Geometry check sheet. Reference: the model listing, model coordinates, mm. Face numbers are marked on the shaded views. A direction names the side the tool comes from. Give positions to 0.01 mm unless a question says otherwise; leave off trailing zeros. Loops run counter-clockwise (first coordinate to the right, second up) from the corner with the lowest first, then second, coordinate; pieces in that order, holes last. Notation, with made-up numbers: (87, 18) -> (122, 18) arc R22 cw to (122, 49) -> close; hole circle Ø10 at (-3.5, -32). An arc over 180 degrees is marked (long way). One line per question, with ' | ' between items.
from build123d import *

# Parameters (mm, degrees)
F0_R     = 1.5
F1_DEPTH = 8
F2_W     = 14.905
F2_H     = 7.65
F3_DEPTH = 7.001
F4_W     = 10.16
F4_H     = 12.091013
F5_DEPTH = 8.351


with BuildPart() as f1:
    # F0 (on Front) → F1 (new body, symmetric)
    with BuildSketch(Plane.XZ):
        with BuildLine():
            Line((9.825, 3.5), (-9.825, 3.5))
            ThreePointArc((-9.825, 3.5), (-13.325, 0), (-9.825, -3.5))
            Line((-9.825, -3.5), (9.825, -3.5))
            ThreePointArc((9.825, -3.5), (13.325, 0), (9.825, 3.5))
        make_face()
        with Locations((-9.825, 0)):
            Circle(F0_R, mode=Mode.SUBTRACT)
        with Locations((9.825, 0)):
            Circle(F0_R, mode=Mode.SUBTRACT)
    extrude(amount=F1_DEPTH, both=True)

    # F2 (on face) → F3 (cut, through all)
    with BuildSketch(Plane.XY.offset(3.5)):
        Polygon((27.112617, -0.35), (9.825, -0.35), (9.825, -8), (-5.08, -8), (-5.08, -17.684488), (27.112617, -17.684488), align=None)
        with Locations((2.3725, -4.175)):
            Rectangle(F2_W, F2_H)
    extrude(amount=-F3_DEPTH, mode=Mode.SUBTRACT)

    # F4 (on face) → F5 (cut, through all)
    with BuildSketch(Plane.XZ.offset(0.35)):
        with Locations((0, 6.045507)):
            Rectangle(F4_W, F4_H)
    extrude(amount=-F5_DEPTH, mode=Mode.SUBTRACT)


solid = f1.part
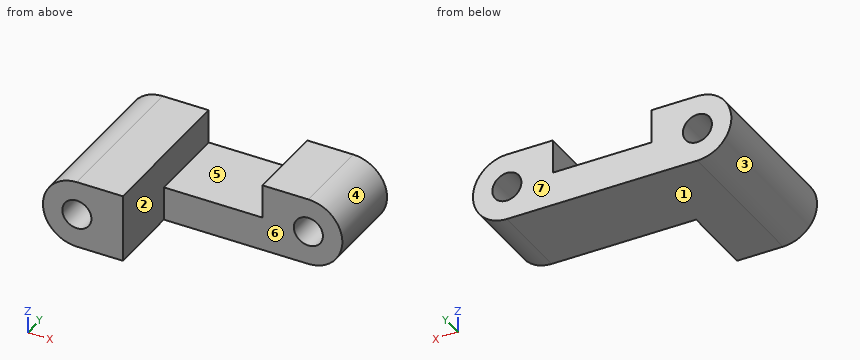
Item 1: Sectioned sample at C-C (z = -0.75). Record the cut outline in (x, y).
Result:
outline: (-13.24, -8) -> (-11.12, -8) -> (-11.12, 8) -> (-13.24, 8) -> close; (-8.53, -8) -> (-5.08, -8) -> (-5.08, -0.35) -> (8.53, -0.35) -> (8.53, 8) -> (-8.53, 8) -> close; (11.12, -0.35) -> (13.24, -0.35) -> (13.24, 8) -> (11.12, 8) -> close
Item 2: Sectioned sample at A-A (y = 0.75). Record the cut outline in (x, z) (3 decimals), plus the area to 3 significant figures.
Result:
outline: (-9.825, -3.5) -> (9.825, -3.5) arc R3.5 ccw to (9.825, 3.5) -> (5.08, 3.5) -> (5.08, 0) -> (-5.08, 0) -> (-5.08, 3.5) -> (-9.825, 3.5) arc R3.5 ccw to start; hole circle Ø3 at (-9.825, 0); hole circle Ø3 at (9.825, 0) | area: 126 mm2
Item 3: Sectioned sample at B-B (z = 2.25). Record the cut outline in (x, y).
Result:
outline: (-12.51, -8) -> (-5.08, -8) -> (-5.08, 8) -> (-12.51, 8) -> close; (5.08, -0.35) -> (12.51, -0.35) -> (12.51, 8) -> (5.08, 8) -> close
Item 4: Scan lines: probe 1 along X at (y, z) = (7.25, 0.5); probe 2 along Y at (x, z) = (5.5, -0.75); probe 3 along Z at (x, y) = (-4.5, 1.25). Record each from-to range of solid material in increasing order.
Result:
probe 1: -13.29 to -11.24, -8.41 to -5.08, 5.08 to 8.41, 11.24 to 13.29 | probe 2: -0.35 to 8 | probe 3: -3.5 to 0
Item 5: Set-up check for the marked faces 5, 6 and 7: record each of +Z, -Z, +X, -X, +Y, -Y from which the full face is reachable in a straight line by a thin tool's end or side.
Result:
face 5: +Z, +Y, -Y | face 6: +Z, -Z, +X, -Y | face 7: +Z, -Z, +X, -X, +Y
Item 6: Sectioned sample at D-D (y = -4.5). Record the cut outline in (x, z) (3 decimals), plus the area to 3 significant figures.
Result:
outline: (-9.825, -3.5) -> (-5.08, -3.5) -> (-5.08, 3.5) -> (-9.825, 3.5) arc R3.5 ccw to start; hole circle Ø3 at (-9.825, 0) | area: 45.4 mm2
Item 7: Release check for a two-part mould opening along X. For the marked faces 1, 2, 3 and 4 record: pulls with the +X half, pulls with the -X half, needs draft (parallel to the pull), parting line crosses it, or undercut.
Result:
face 1: needs draft | face 2: undercut | face 3: pulls with the -X half | face 4: pulls with the +X half
Item 8: Depth check by flat-ended pin: pin 1 Ø1 at (y, z) = (4.5, 2) entering from -X; pin 2 Ø3.5 at (y, z) = (-2, -1) entering from +X; pin 3 Ø1 at (y, z) = (2, 3) entering from +X. Enter the tip coordinate at first touch or a pass-through.
Result:
pin 1: x = -12.99 | pin 2: x = 13.3 | pin 3: x = 12.27
